from build123d import *

# Parameters (mm, degrees)
F0_R     = 1.849397
F1_DEPTH = 2.2


with BuildPart() as f1:
    # F0 (on Top) → F1 (new body)
    with BuildSketch(Plane.XY):
        with BuildLine():
            ThreePointArc((-43.155712, 41.621163), (-49.121705, 48.332393), (-55.155712, 41.682247))
            Line((-55.155712, 41.682247), (-50.748931, 19.573376))
            ThreePointArc((-50.748931, 19.573376), (-49.15236, 19.55101), (-47.555789, 19.573379))
            Line((-47.555789, 19.573379), (-43.155712, 41.621163))
        make_face()
        with Locations((-49.152423, 42.297715)):
            Circle(F0_R, mode=Mode.SUBTRACT)
        with BuildLine():
            ThreePointArc((-47.555789, 19.573379), (-49.15236, 19.55101), (-50.748931, 19.573376))
            ThreePointArc((-50.748931, 19.573376), (-54.461987, 19.798882), (-58.152423, 20.266136))
            ThreePointArc((-58.152423, 20.266136), (-49.152423, 5.217745), (-40.152423, 20.266136))
            ThreePointArc((-40.152423, 20.266136), (-43.842796, 19.798888), (-47.555789, 19.573379))
        make_face()
    extrude(amount=F1_DEPTH)


solid = f1.part
Could you check a few things on this model? Use its own coordinates, in mm. A direction names the side the tool comes from. Coordinates: 2 decimals unless noted, no trailing zeros. Order: outer loops, then holes, each group sorted by start corner. A loop starts at its lowest first (then second) coordinate and runs counter-clockwise, first axis right, second up.
Q1. Suppose I cut it at A-A on x = -54.5. Please give me the cut outline in (y, z).
Q2. Suppose I cut it at D-D on y = 28. Please give me the cut outline in (x, z), and give its area (3 significant figures).
Q3. Thinking about a two-plate mould opening in X: for faces 1 (the flat face through (-49, 22, 0)), 2 (the cylindrical face through (-48.98, 48.33, 1.08)), 3 (the cylindrical face through (-47.388, 42.853, 1.085)), which applies, released by +X, released by -X, zero draft, split by the parting line, or undercut?
Q4. Please list where these lines run through material, in increasing order: L1, parallel to X at y = 23, z = 1.35; L2, parallel to X at y = 25, z = 1.6; L3, parallel to Y at x = -57.5, z = 1.
Q5. Which directions (+Z, -Z, +X, -X, +Y, -Y) give clear straight access to the entire face, cutting with the end or side of a thin tool? Please do faces 4 (the flat face through (-49, 22, 2.2)), 5 (the cylindrical face through (-43.791, 19.804, 1.085)).
Q6. Suppose I cut it at B-B on z = 1.1. Please give me the cut outline in (x, y), and give its area (3 significant figures).
Q7. Suppose I cut it at C-C on x = -49.5. Please give me the cut outline in (y, z).
Answer:
1. outline: (6.73, 0) - (19.8, 0) - (19.8, 2.2) - (6.73, 2.2) - close; (38.39, 0) - (45.09, 0) - (45.09, 2.2) - (38.39, 2.2) - close
2. outline: (-52.43, 0) - (-45.87, 0) - (-45.87, 2.2) - (-52.43, 2.2) - close
2. area: 14.4 mm2
3. face 1: zero draft
3. face 2: split by the parting line
3. face 3: undercut
4. L1: x = -51.43 to -46.87
4. L2: x = -51.83 to -46.47
4. L3: y = 9.54 to 20.17
5. face 4: +Z, +X, -X, +Y, -Y
5. face 5: +Z, -Z
6. outline: (-58.15, 20.27) arc R10.22 ccw (long way) to (-40.15, 20.27) arc R56.99 cw to (-47.56, 19.57) - (-43.16, 41.62) arc R6.03 ccw (long way) to (-55.16, 41.68) - (-50.75, 19.57) arc R56.99 cw to start; hole circle Ø3.7 at (-49.15, 42.3)
6. area: 472 mm2
7. outline: (5.22, 0) - (40.48, 0) - (40.48, 2.2) - (5.22, 2.2) - close; (44.11, 0) - (48.32, 0) - (48.32, 2.2) - (44.11, 2.2) - close
